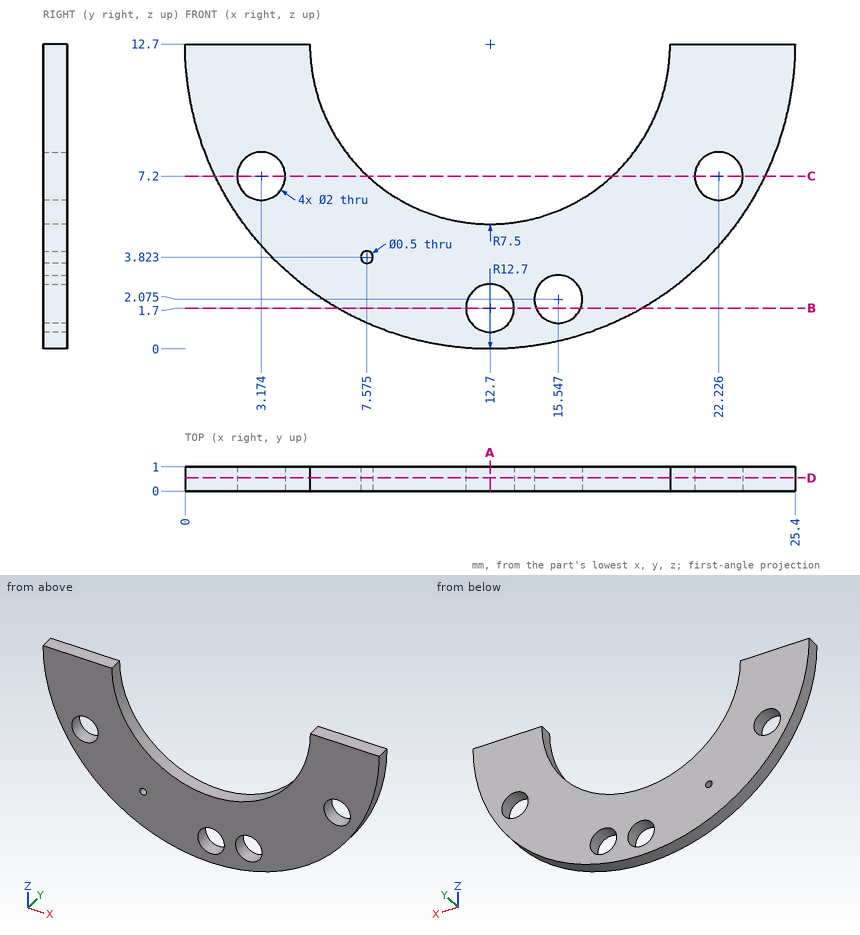
Geometry: see drawing. Coordinates: mm, zero at the bounding-box minimum. Coordinates: 2 decimals unless noted, no trailing zeros. Loops run counter-clockwise (first coordinate to the right, second up) from the corner with the lowest first, then second, coordinate; pieces in that order, holes last. Notation, with made-up numbers: M -23.75,73.5 L -0.75,73.5 A16 cw -0.75,81.5 Z; hole C -35.75,40 d3. An arc over 180 degrees is marked long. Answer in a Markdown table with one row per item.
1. First-contact query: pin 1 (1.8 mm diameter, centred on x = 12.7, z = 1.7, fed in from +Y). Flat tip, straight axial feed; report the tip coordinate or a pass-through.
Response:
| item | result |
|---|---|
| pin 1 | passes through |
2. Section D-D, the plane y = 0.55. Count the separate pieces of the cut face and the enclosed holes in it, then the cut area to 3 significant figures.
Response:
| item | result |
|---|---|
| separate pieces | 1 |
| enclosed holes | 5 |
| area | 152 mm2 |
3. Section A-A, the plane x = 12.7. Output: boundary loops of the cut face in (y, z).
Response:
| item | result |
|---|---|
| outline | M 0,0 L 1,0 L 1,0.7 L 0,0.7 Z; M 0,2.7 L 1,2.7 L 1,5.2 L 0,5.2 Z |
4. Section C-C, the plane z = 7.2. Output: boundary loops of the cut face in (x, y).
Response:
| item | result |
|---|---|
| outline | M 1.25,0 L 2.17,0 L 2.17,1 L 1.25,1 Z; M 4.17,0 L 7.6,0 L 7.6,1 L 4.17,1 Z; M 17.8,0 L 21.23,0 L 21.23,1 L 17.8,1 Z; M 23.23,0 L 24.15,0 L 24.15,1 L 23.23,1 Z |
5. Section B-B, the plane z = 1.7. Output: boundary loops of the cut face in (x, y).
Response:
| item | result |
|---|---|
| outline | M 6.35,0 L 11.7,0 L 11.7,1 L 6.35,1 Z; M 13.7,0 L 14.62,0 L 14.62,1 L 13.7,1 Z; M 16.47,0 L 19.05,0 L 19.05,1 L 16.47,1 Z |
6. Material intervals for line 1 (X direction, y = 0.75, z = 7.2) (1 decimal); line 2 (Z direction, x = 12.7, y = 0.3); line 3 (X direction, y = 0.2, z = 10), sorted ascending.
Response:
| item | result |
|---|---|
| line 1 | x = 1.3 to 2.2, 4.2 to 7.6, 17.8 to 21.2, 23.2 to 24.1 |
| line 2 | z = 0 to 0.7, 2.7 to 5.2 |
| line 3 | x = 0.29 to 5.7, 19.7 to 25.11 |
